Verification items for the finished model (mm, model axes). Face numbers are marked on the shaded views. A direction names the side the tool comes from. Round coordinates to 2 decimals unless told otherwise and drop trailing zeros. Order: outer loops, then holes, each group sorted by start corner. A loop starts at its lowest first (then second) coordinate and runs counter-clockwise, first axis right, second up. Notation, with made-up numbers: (52, -4) -> (73, -4) arc R18 ccw to (73, 0) -> close; hole circle Ø1 at (65.5, -2). An arc over 180 degrees is marked (long way). Return JSON: item names as keys, results as strings. Group by question number.
Item 1: Sectioned sample at A-A on y = 32.5. Record the cut outline in (x, z).
Item 2: Access from +Z, -Z, +X, -X, +Y, -Y to the whole of each face (thin tool, end or side, straight path). Record for the marked faces 5 and 6.
Item 3: Sectioned sample at B-B on x = -14. Record the cut outline in (y, z).
Item 4: Scan lines: probe 1 along Z at (x, y) = (-9, -36); probe 2 along Z at (x, y) = (31.3, 18.5); probe 3 along X at (y, z) = (43.5, -7.5). Record each from-to range of solid material in increasing order. Write a range as from..to.
Item 5: Draft check along Z on the marked faces 1, 2, 3 and 4. Enter one of: pulls with the +Z half, pulls with the -Z half, needs draft (parallel to the pull), parting line crosses it, or undercut.
Item 6: Depth check by flat-ended pin: pin 1 Ø1.8 at (x, z) = (-31.3, 0) entering from +Y; pin 2 Ø2 at (y, z) = (-42, -4.5) entering from +X; pin 3 Ø8 at (y, z) = (0, -4.5) entering from +X; pin 4 Ø2 at (y, z) = (-25.5, -2) entering from -X. Enter the tip coordinate at first touch or a pass-through.
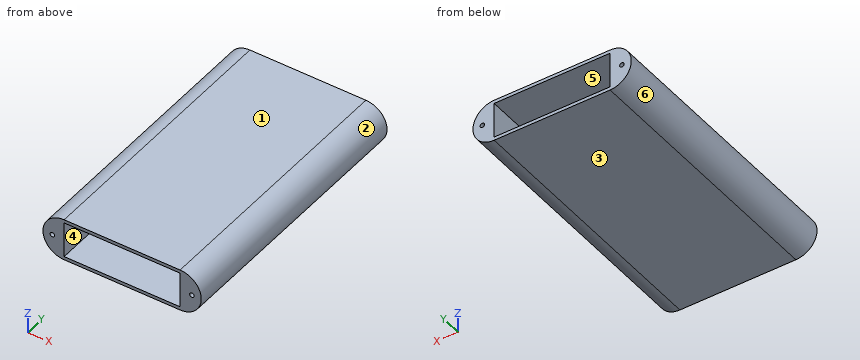
```python
from build123d import *

# Parameters (mm, degrees)
BOSS_EXTRUDE1_DEPTH = 60.5
SHELL1_T            = -1.5
BOSS_EXTRUDE2_DEPTH = 60.5


with BuildPart() as part:
    # Sketch1 → Boss-Extrude1 (new, symmetric)
    with BuildSketch(Plane(origin=(0, 0, 0), x_dir=(1, 0, 0), z_dir=(0, 1, 0))):
        with BuildLine():
            Line((-26, 9.5), (26, 9.5))
            ThreePointArc((26, 9.5), (35.5, 0), (26, -9.5))
            Line((26, -9.5), (-26, -9.5))
            ThreePointArc((-26, -9.5), (-35.5, 0), (-26, 9.5))
        make_face()
    extrude(amount=BOSS_EXTRUDE1_DEPTH, both=True)

    # Shell1
    shell1_openings = [part.faces().sort_by_distance(p)[0] for p in [
        (0, 60.5, 0),
        (0, -60.5, 0),
    ]]
    offset(amount=SHELL1_T, openings=shell1_openings, kind=Kind.INTERSECTION)

    # Sketch2 → Boss-Extrude2 (add, symmetric)
    with BuildSketch(Plane(origin=(0, 0, 0), x_dir=(1, 0, 0), z_dir=(0, 1, 0))):
        with BuildLine():
            ThreePointArc((-34, 0), (-31.656854249, -5.656854249), (-26, -8))
            Line((-26, -8), (-26, 0))
            Line((-26, 0), (-30.3, 0))
            ThreePointArc((-30.3, 0), (-31.3, -1), (-32.3, 0))
            Line((-32.3, 0), (-34, 0))
        make_face()
        with BuildLine():
            Line((-30.3, 0), (-26, 0))
            Line((-26, 0), (-26, 8))
            ThreePointArc((-26, 8), (-31.656854249, 5.656854249), (-34, 0))
            Line((-34, 0), (-32.3, 0))
            ThreePointArc((-32.3, 0), (-31.3, 1), (-30.3, 0))
        make_face()
    boss_extrude2 = extrude(amount=BOSS_EXTRUDE2_DEPTH, both=True)

    # Mirror1: Boss-Extrude2 across plane
    add(boss_extrude2.mirror(Plane(origin=(0, 0, 0), x_dir=(0, 0, 1), z_dir=(1, 0, 0))))


solid = part.part
```
Recorded:
{
 "1": {"outline": "(-26, -9.5) -> (26, -9.5) arc R9.5 ccw to (26, 9.5) -> (-26, 9.5) arc R9.5 ccw to start; hole circle Ø2 at (-31.3, 0); hole (-26, -8) -> (26, -8) -> (26, 8) -> (-26, 8) -> close; hole circle Ø2 at (31.3, 0)"},
 "2": {"face 5": "+Y, -Y", "face 6": "-X, +Y, -Y"},
 "3": {"outline": "(-60.5, -9.5) -> (60.5, -9.5) -> (60.5, -8) -> (-60.5, -8) -> close; (-60.5, 8) -> (60.5, 8) -> (60.5, 9.5) -> (-60.5, 9.5) -> close"},
 "4": {"probe 1": "-9.5..-8, 8..9.5", "probe 2": "-7.88..-1, 1..7.88", "probe 3": "-31.83..-26, 26..31.83"},
 "5": {"face 1": "pulls with the +Z half", "face 2": "parting line crosses it", "face 3": "pulls with the -Z half", "face 4": "undercut"},
 "6": {"pin 1": "through", "pin 2": "x = 34.83", "pin 3": "x = 35.49", "pin 4": "x = -35.45"}
}
